Answer from the drawing. Dimensions are ordinates in mm from the lowest x, y and z of the part. Coordinates: 2 decimals unless noted, no trailing zeros. Write each loop counter-clockwise with the first axis right and the second up, starting at its lowest first coordinate (ties: lowest second). Pieces come first, ordered by that corner, then holes.
1) Find the intervals of material crossed by line 1 (Y direction, x = 87, z = 2.05); line 2 (X direction, y = 13, z = 2.3); line 3 (Z direction, x = 94.5, y = 2.5), in increasing order.
2) The part is cut by section A-A (z = 2.8). Determine the outline of the cut face in (x, y).
3) This flat-tipped pin is pushed along its axis until it touches: pin 1 Ø6 at (x, y) = (80.5, 37.5) entering from +Z. Where does it stop, or does it pass through?
4) The part is cut by section B-B (x = 48). Determine the outline of the cut face in (y, z).
5) Determine the mould class of the marked faces 1 and 2 for opening direction X: +X half, -X half, draft (parallel to the pull), parting line (faces both ways), or undercut.
6) The part is cut by section C-C (y = 6). Determine the outline of the cut face in (x, z).
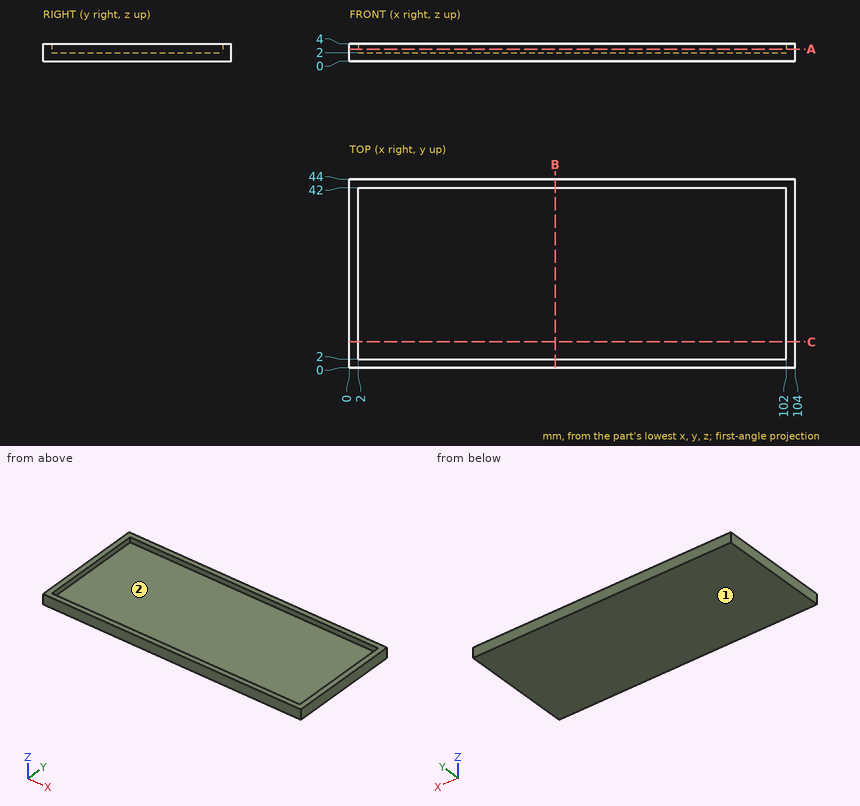
Reported:
1. line 1: y = 0 to 2, 42 to 44
1. line 2: x = 0 to 2, 102 to 104
1. line 3: z = 0 to 2
2. outline: (0, 0) - (104, 0) - (104, 44) - (0, 44) - close; hole (2, 2) - (102, 2) - (102, 42) - (2, 42) - close
3. pin 1: stops at z = 2
4. outline: (0, 0) - (44, 0) - (44, 4) - (42, 4) - (42, 2) - (2, 2) - (2, 4) - (0, 4) - close
5. face 1: draft
5. face 2: undercut
6. outline: (0, 0) - (104, 0) - (104, 4) - (102, 4) - (102, 2) - (2, 2) - (2, 4) - (0, 4) - close
